Study the drawing (mm; zero at the part's minimum x, y, z) and answer. Coordinates: 2 decimals unless noted, no trailing zeros. Loops run counter-clockwise (first coordinate to the right, second up) from the corner with the lowest first, then second, coordinate; pieces in that order, holes last. Notation, with made-up numbers: (35.25, 45.5) - (60.25, 45.5) arc R16 cw to (60.25, 74.5) - close; hole circle Ø2 at (54.5, -40). An arc over 180 degrees is marked (long way). Use CSV: the item, a comma, the result in double quotes.
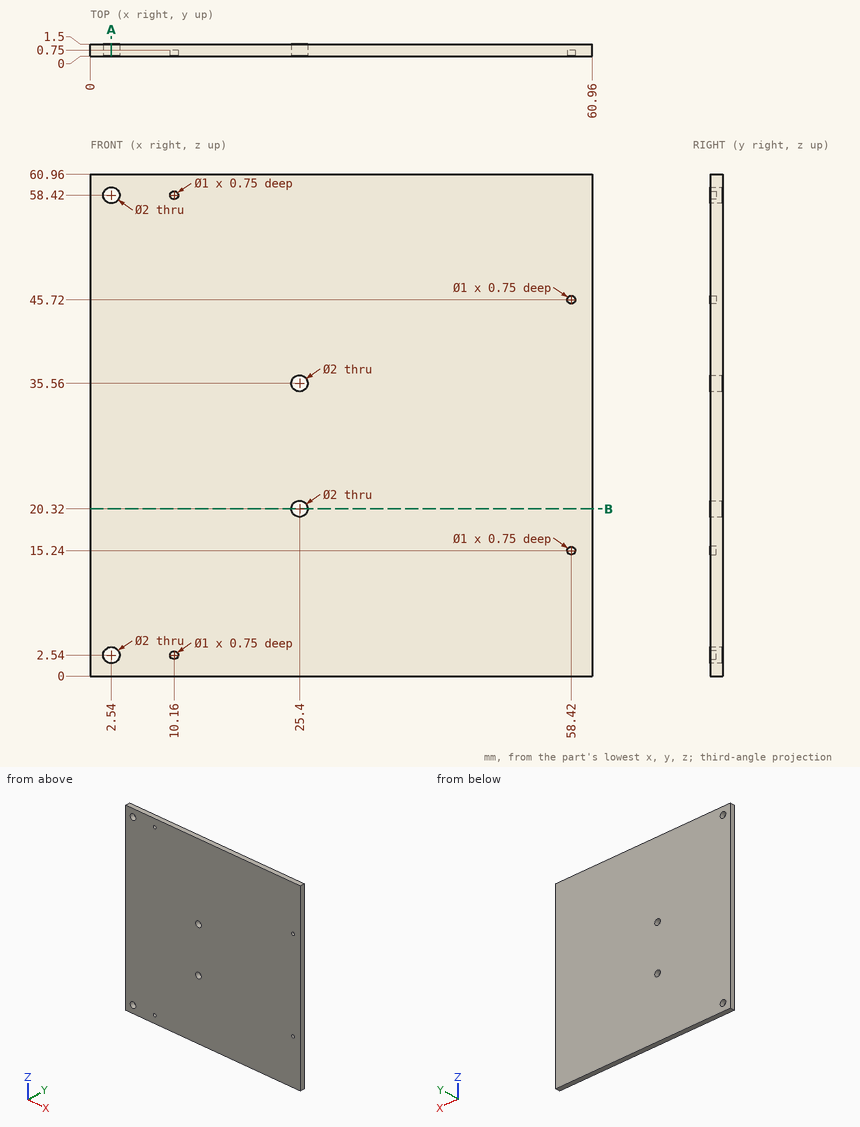
Q1. The part is cut by section B-B on z = 20.32. Determine the outline of the cut face in (x, y), and give its area (3 significant figures).
Reported:
outline,"(0, 0) - (24.4, 0) - (24.4, 1.5) - (0, 1.5) - close; (26.4, 0) - (60.96, 0) - (60.96, 1.5) - (26.4, 1.5) - close"
area,"88.4 mm²"
Q2. Find the intervals of material crossed by probe 1 along Z at (x, y) = (58.42, 0.55); probe 2 along X at (y, z) = (0.3, 58.42); probe 3 along X at (y, z) = (0.8, 20.32), in increasing order. Write a range as [from, to].
Reported:
probe 1,"z = [0, 14.74], [15.74, 45.22], [46.22, 60.96]"
probe 2,"x = [0, 1.54], [3.54, 9.66], [10.66, 60.96]"
probe 3,"x = [0, 24.4], [26.4, 60.96]"
Q3. Given P1, Ø1.2, axis at x = 2.54, z = 2.54, coming from the +Y side, flat-ended and moving along its own axis, determine where the tip first touches the part or whether it passes through.
Reported:
P1,"passes through"
Q4. The part is cut by section A-A on x = 2.54. Determine the outline of the cut face in (y, z).
Reported:
outline,"(0, 0) - (1.5, 0) - (1.5, 1.54) - (0, 1.54) - close; (0, 3.54) - (1.5, 3.54) - (1.5, 57.42) - (0, 57.42) - close; (0, 59.42) - (1.5, 59.42) - (1.5, 60.96) - (0, 60.96) - close"
